Job drawing, mm, ordinate dimensions from the low corner. One solid piece. A direction names the side the tool comes from. Coordinates: 2 decimals unless noted, no trailing zeros. Loops run counter-clockwise (first coordinate to the right, second up) from the corner with the lowest first, then second, coordinate; pieces in that order, holes last. Notation, with made-up numbers: (-6, 54) -> (5, 54) arc R15 cw to (5, 60) -> close; hole circle Ø11 at (-11, 35). An arc over 180 degrees is marked (long way). Use one line per item in the form item = value. Start each with the question number.
(1) Mould opens along X. For the marked faces 1, 2 and 3 say: +X half, -X half, draft (parallel to the pull), parting line (faces both ways), or undercut.
(2) Band-saw the part on C-C on y = 4. Give the cut face in (x, z).
(3) Band-saw the part on A-A on z = 19.5. Give the cut face in (x, y), then the cut area to 3 significant figures.
(4) Drill centre lines: L1, parallel to Y at x = 2, z = 9.25; L2, parallel to X at y = 2, z = 14; L3, parallel to Z at x = 20.5, y = 5. Where is each one in solid material? Low to high. Write a range as [from, to].
(5) 3-axis set-ups, long thin cutter, end or side, ignore diameter. For the marked faces 4, 5 and 6: which of +Z, -Z, +X, -X, +Y, -Y reach the whole face in a straight line?
(6) Band-saw the part on D-D on z = 6. Give the cut face in (x, y), then the cut area to 3 significant figures.
(7) Pin check, flat tips, straight feed: P1, Ø12, axis at x = 7, z = 12, coming from the -Y side; P2, Ø4, axis at x = 4.5, z = 8.5, coming from the +Y side; P3, Ø1.2, axis at y = 9.5, z = 1.5, coming from the +X side; P4, Ø0.5, axis at x = 0.5, y = 4, coming from the +Z side. Stop position of each tip, or through.
(8) Band-saw the part on B-B on x = 7.75. Give the cut face in (y, z), then the cut area to 3 significant figures.
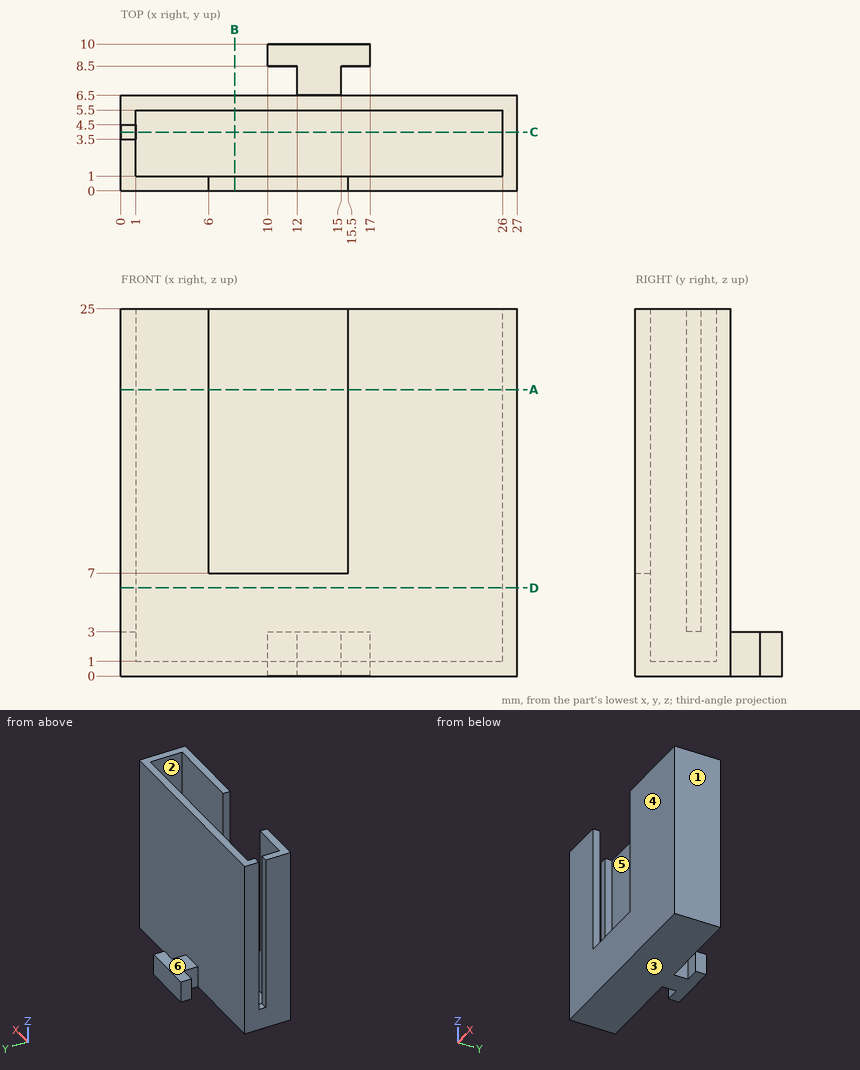
A:
q1.face_1 = +X half
q1.face_2 = undercut
q1.face_3 = draft
q2.outline = (0, 0) -> (27, 0) -> (27, 25) -> (26, 25) -> (26, 1) -> (1, 1) -> (1, 3) -> (0, 3) -> close
q3.outline = (0, 0) -> (6, 0) -> (6, 1) -> (1, 1) -> (1, 3.5) -> (0, 3.5) -> close; (0, 4.5) -> (1, 4.5) -> (1, 5.5) -> (26, 5.5) -> (26, 1) -> (15.5, 1) -> (15.5, 0) -> (27, 0) -> (27, 6.5) -> (0, 6.5) -> close
q3.area = 52.5 mm²
q4.L1 = [0, 1], [5.5, 6.5]
q4.L2 = [0, 1], [26, 27]
q4.L3 = [0, 1]
q5.face_4 = +Z, -Z, +X, -X, -Y
q5.face_5 = +Z
q5.face_6 = +Z, +X, -X, +Y
q6.outline = (0, 0) -> (27, 0) -> (27, 6.5) -> (0, 6.5) -> (0, 4.5) -> (1, 4.5) -> (1, 5.5) -> (26, 5.5) -> (26, 1) -> (1, 1) -> (1, 3.5) -> (0, 3.5) -> close
q6.area = 62.0 mm²
q7.P1 = 0
q7.P2 = 6.5
q7.P3 = 17
q7.P4 = 3
q8.outline = (0, 0) -> (6.5, 0) -> (6.5, 25) -> (5.5, 25) -> (5.5, 1) -> (1, 1) -> (1, 7) -> (0, 7) -> close
q8.area = 36.5 mm²
